The figure shows three views and two pictorial views of one solid part (mm, origin at its lowest corner). Answer the questions. Round coordinates to 2 decimals unless told otherwise and drop trailing zeros. Order: outer loops, then holes, each group sorted by start corner. A loop starts at its lowest first (then second) coordinate and runs counter-clockwise, first axis right, second up. Notation, with made-up numbers: (27, -37.5) - (31, -37.5) arc R29 ccw to (31, -9.5) - close; hole circle Ø7 at (-32.75, 59). An arc over 180 degrees is marked (long way). One line per item, written item: value. Start each with the question number.
1. Section A-A, the plane x = 21.59 is taken. Give the vertices of the cut face in (y, z) (1 decimal).
2. Section B-B, the plane z = 7.25 is taken. Give the vertices of the cut face in (x, y).
3. Section D-D, the plane y = 1 is taken. Give the vertices of the cut face in (x, z).
4. Section C-C, the plane y = 7 is taken. Count the separate pieces of the cut face and the enclosed holes in it, then the cut area to 3 significant figures.
5. Straight lines are drawn through the part: line 1 (X direction, y = 6.25, z = 11.25); line 2 (X direction, y = 6.75, z = 5.5); line 3 (Z direction, x = 82.55, y = 2.5) (1 decimal). For each, find the intervals that lie inside material, in ascending order.
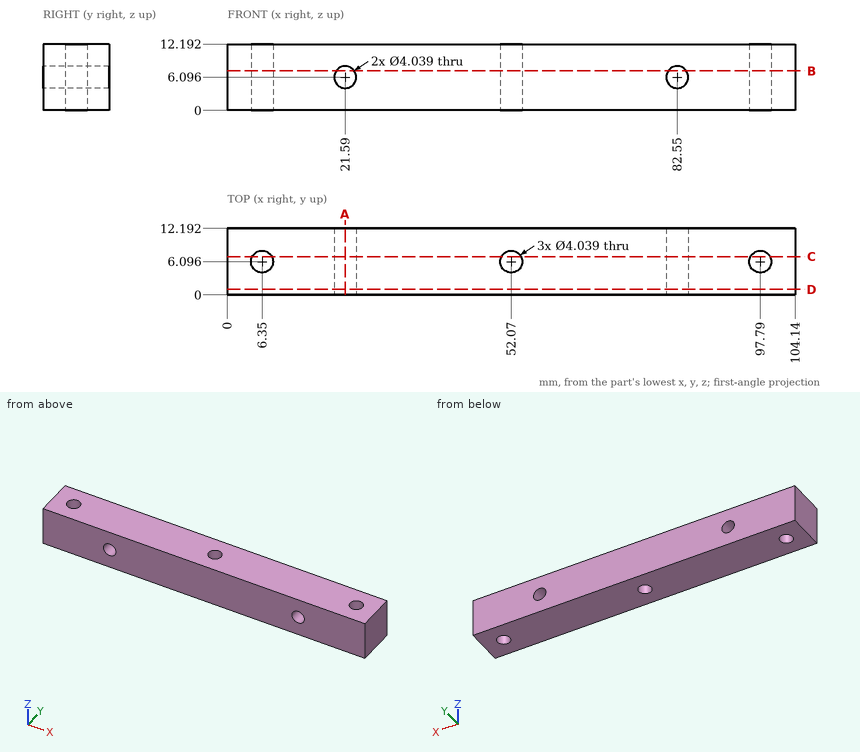
Answer list:
1. outline: (0, 0) - (12.2, 0) - (12.2, 4.1) - (0, 4.1) - close; (0, 8.1) - (12.2, 8.1) - (12.2, 12.2) - (0, 12.2) - close
2. outline: (0, 0) - (19.93, 0) - (19.93, 12.19) - (0, 12.19) - close; (23.25, 0) - (80.89, 0) - (80.89, 12.19) - (23.25, 12.19) - close; (84.21, 0) - (104.14, 0) - (104.14, 12.19) - (84.21, 12.19) - close; hole circle Ø4.04 at (6.35, 6.1); hole circle Ø4.04 at (52.07, 6.1); hole circle Ø4.04 at (97.79, 6.1)
3. outline: (0, 0) - (104.14, 0) - (104.14, 12.19) - (0, 12.19) - close; hole circle Ø4.04 at (21.59, 6.1); hole circle Ø4.04 at (82.55, 6.1)
4. separate pieces: 4
4. enclosed holes: 2
4. area: 1,110 mm²
5. line 1: x = 0 to 4.34, 8.36 to 50.06, 54.08 to 95.78, 99.8 to 104.14
5. line 2: x = 0 to 4.44, 8.26 to 19.66, 23.52 to 50.16, 53.98 to 80.62, 84.48 to 95.88, 99.7 to 104.14
5. line 3: z = 0 to 4.1, 8.1 to 12.2
